Read the model definition and answer for the solid it produces. Units are mm, in the model's axes. A direction names the side the tool comes from. Give positions to 0.01 mm unless a question says otherwise; leave off trailing zeros. Loops run counter-clockwise (first coordinate to the right, second up) from the corner with the lowest first, then second, coordinate; pieces in that order, holes last. Notation, with made-up numbers: (-39, 22.25) - (-28, 22.25) arc R10 cw to (-28, 32.25) - close; hole circle Ø10 at (34.25, -17.75). An arc over 180 degrees is marked (long way). Use a Markdown table: item, result. Add a question column.
Item 1: A cutting plane is placed at B-B (z = -24). Determine the outline of the cut face in (x, y).
Item 2: For a pull along Z with two mould halves and no side action, classify faces 5 (the face through (-24.89, 6.93, -19.64)), 6 (the face through (-25, 4, 28)), 7 (the face through (-15, -2, 0)) as +Z half, -Z half, draft (parallel to the pull), parting line (faces both ways), or undercut.
Item 3: A cutting plane is placed at C-C (x = -30). Determine the outline of the cut face in (y, z).
Item 4: Which of the six approach directions +Z, -Z, +X, -X, +Y, -Y give full straight-line access (tool end or side, diameter ignored) to faces 1 (the face through (-25, 7, 31)), 2 (the face through (-14.68, 4, 32)), 3 (the face through (-33, 7, -3)), 4 (the face through (15, 7, 31))?
Item 5: A cutting plane is placed at A-A (y = 5.5). Determine the outline of the cut face in (x, z).
Item 6: Each of these flat-tipped pins is pushed along its axis until it touches: P1, Ø8, axis at x = -9.5, z = 2, coming from the +Y side; P2, Ø1.8, axis at x = -13, y = 5.5, coming from the +Z side; P3, Ø5, axis at x = 30, z = -24, coming from the -Y side; P4, Ø5.5, axis at y = 4.5, z = 30, coming from the +X side. Where does it stop, or does it pass through?
Item 7: Consider probe 1 along X at (y, z) = (1, -24); probe 2 along Y at (x, z) = (-13, -30); probe 3 along Y at (x, z) = (-15, -28). Determine where each line is inside the solid, lowest interval first. Write a range as [from, to].
Item 8: A cutting plane is placed at D-D (z = -11). Determine the outline of the cut face in (x, y).
from build123d import *

# Parameters (mm, degrees)
SKIZZE1_W                       = 70
SKIZZE1_H                       = 70
SKIZZE1_R                       = 1.5
AUFSATZ_LINEAR_AUSTRAGEN1_DEPTH = 2
SKIZZE2_W                       = 20.32
SKIZZE2_H                       = 7
AUFSATZ_LINEAR_AUSTRAGEN2_DEPTH = 5
AUFSATZ_LINEAR_AUSTRAGEN3_DEPTH = 10
SKIZZE4_W                       = 30
SKIZZE4_H                       = 30
AUFSATZ_LINEAR_AUSTRAGEN4_DEPTH = 10
SKIZZE5_R                       = 2.5
SKIZZE5_R_2                     = 1.5
AUFSATZ_LINEAR_AUSTRAGEN5_DEPTH = 10
SKIZZE6_W                       = 25
SKIZZE6_H                       = 25
AUFSATZ_LINEAR_AUSTRAGEN6_DEPTH = 3.5
VERRUNDUNG1_R                   = 3


with BuildPart() as part:
    # Skizze1 → Aufsatz-Linear austragen1 (new body)
    with BuildSketch(Plane(origin=(0, 0, 0), x_dir=(1, 0, 0), z_dir=(0, 1, 0))):
        Rectangle(SKIZZE1_W, SKIZZE1_H)
        with Locations((-6, -31)):
            Circle(SKIZZE1_R, mode=Mode.SUBTRACT)
        with Locations((-30, 24)):
            Circle(SKIZZE1_R, mode=Mode.SUBTRACT)
        with Locations((30, 24)):
            Circle(SKIZZE1_R, mode=Mode.SUBTRACT)
    extrude(amount=AUFSATZ_LINEAR_AUSTRAGEN1_DEPTH)

    # Skizze2 → Aufsatz-Linear austragen2 (add)
    with BuildSketch(Plane(origin=(0, 2, 0), x_dir=(1, 0, 0), z_dir=(0, 1, 0))):
        with Locations((-24.84, -31.5)):
            Rectangle(SKIZZE2_W, SKIZZE2_H)
    extrude(amount=AUFSATZ_LINEAR_AUSTRAGEN2_DEPTH)

    # Skizze3 → Aufsatz-Linear austragen3 (add)
    with BuildSketch(Plane(origin=(0, 2, 0), x_dir=(1, 0, 0), z_dir=(0, 1, 0))):
        Polygon((-33, -7.164928148), (-23, -7.164928148), (-3, -31), (33, -31), (33, 21.260665951), (28, 21.260665951), (28, 26.260665951), (-17, 26.260665951), (-33, 12.835071852), align=None)
    extrude(amount=AUFSATZ_LINEAR_AUSTRAGEN3_DEPTH)

    # Skizze4 → Aufsatz-Linear austragen4 (add)
    with BuildSketch(Plane(origin=(0, 12, 0), x_dir=(1, 0, 0), z_dir=(0, 1, 0))):
        with Locations((15.5, -15)):
            Rectangle(SKIZZE4_W, SKIZZE4_H)
    extrude(amount=AUFSATZ_LINEAR_AUSTRAGEN4_DEPTH)

    # Skizze5 → Aufsatz-Linear austragen5 (add)
    with BuildSketch(Plane(origin=(0, 0, -26.260665951), x_dir=(-1, 0, 0), z_dir=(0, 0, -1))):
        with Locations((13, 5.5)):
            Circle(SKIZZE5_R)
        with Locations((13, 5.5)):
            Circle(SKIZZE5_R_2, mode=Mode.SUBTRACT)
    extrude(amount=AUFSATZ_LINEAR_AUSTRAGEN5_DEPTH)

    # Skizze6 → Aufsatz-Linear austragen6 (add)
    with BuildSketch(Plane.XZ):
        with Locations((-14.5, -12.5)):
            Rectangle(SKIZZE6_W, SKIZZE6_H)
    extrude(amount=AUFSATZ_LINEAR_AUSTRAGEN6_DEPTH)

    # Verrundung1
    verrundung1_edges = [part.edges().sort_by_distance(p)[0] for p in [
        (-35, 1, -35),
        (35, 1, -35),
        (35, 1, 35),
    ]]
    fillet(verrundung1_edges, radius=VERRUNDUNG1_R)


solid = part.part
Geometry says:
| question | item | result |
|---|---|---|
| 1 | outline | (-35, 0) - (-31.5, 0) - (-31.5, 2) - (-35, 2) - close; (-28.5, 0) - (-27, 0) - (-27, -3.5) - (-2, -3.5) - (-2, 0) - (28.5, 0) - (28.5, 2) - (28, 2) - (28, 12) - (-19.69, 12) - (-19.69, 2) - (-28.5, 2) - close; (31.5, 0) - (35, 0) - (35, 2) - (31.5, 2) - close |
| 2 | face 5 | -Z half |
| 2 | face 6 | undercut |
| 2 | face 7 | +Z half |
| 3 | outline | (0, -35) - (2, -35) - (2, -25.5) - (0, -25.5) - close; (0, -22.5) - (2, -22.5) - (2, -15.35) - (12, -15.35) - (12, 7.16) - (2, 7.16) - (2, 28) - (7, 28) - (7, 35) - (0, 35) - close |
| 4 | face 1 | +Z, -X, +Y |
| 4 | face 2 | +Z, +Y |
| 4 | face 3 | -Z, -X, +Y |
| 4 | face 4 | +Z, +X, +Y |
| 5 | outline | (-35, 28) - (-14.68, 28) - (-14.68, 35) - (-35, 35) - close; (-33, -12.84) - (-17, -26.26) - (-15.5, -26.26) - (-15.5, -36.26) - (-14.5, -36.26) - (-14.5, -26.26) - (-11.5, -26.26) - (-11.5, -36.26) - (-10.5, -36.26) - (-10.5, -26.26) - (28, -26.26) - (28, -21.26) - (33, -21.26) - (33, 31) - (-3, 31) - (-23, 7.16) - (-33, 7.16) - close |
| 6 | P1 | y = 12 |
| 6 | P2 | z = 20.16 |
| 6 | P3 | y = 0 |
| 6 | P4 | x = 35 |
| 7 | probe 1 | [-35, -31.5], [-28.5, 28.5], [31.5, 35] |
| 7 | probe 2 | [0, 2], [3, 4], [7, 8] |
| 7 | probe 3 | [0, 2], [4, 7] |
| 8 | outline | (-35, 0) - (-27, 0) - (-27, -3.5) - (-2, -3.5) - (-2, 0) - (35, 0) - (35, 2) - (33, 2) - (33, 12) - (-33, 12) - (-33, 2) - (-35, 2) - close |
